```python
from build123d import *

# Parameters (mm, degrees)
F1_DEPTH      = 50
F1_DEPTH_BACK = 50
F2_T          = -5
F3_R          = 2.5
F4_DEPTH      = 5
F5_R          = 5
F5_R_2        = 2.5
F6_DEPTH      = 3


with BuildPart() as f1:
    # F0 (on Front) → F1 (new body, two sides)
    with BuildSketch(Plane.XZ) as f1_sk:
        Polygon((-50, 0), (50, 0), (60, 33.947153), (-60, 33.947153), align=None)
    extrude(amount=F1_DEPTH)
    extrude(f1_sk.sketch, amount=-F1_DEPTH_BACK)

    # F2
    f2_openings = [f1.faces().sort_by_distance(p)[0] for p in [
        (0, 0, 33.947153),
    ]]
    offset(amount=F2_T, openings=f2_openings)

    # F3 (on face) → F4 (cut, through all)
    with BuildSketch(Plane.XY.offset(5)):
        with Locations((-40, 40)):
            Circle(F3_R)
        with Locations((-40, -40)):
            Circle(F3_R)
        with Locations((40, -40)):
            Circle(F3_R)
        with Locations((40, 40)):
            Circle(F3_R)
    extrude(amount=-F4_DEPTH, mode=Mode.SUBTRACT)

    # F5 (on face) → F6 (cut)
    with BuildSketch(Plane(origin=(0, 0, 0), x_dir=(1, 0, 0), z_dir=(0, 0, -1))):
        with Locations((-40, 40)):
            Circle(F5_R)
        with Locations((-40, 40)):
            Circle(F5_R_2, mode=Mode.SUBTRACT)
        with Locations((40, 40)):
            Circle(F5_R)
        with Locations((40, 40)):
            Circle(F5_R_2, mode=Mode.SUBTRACT)
        with Locations((40, -40)):
            Circle(F5_R)
        with Locations((40, -40)):
            Circle(F5_R_2, mode=Mode.SUBTRACT)
        with Locations((-40, -40)):
            Circle(F5_R)
        with Locations((-40, -40)):
            Circle(F5_R_2, mode=Mode.SUBTRACT)
    extrude(amount=-F6_DEPTH, mode=Mode.SUBTRACT)


solid = f1.part
```
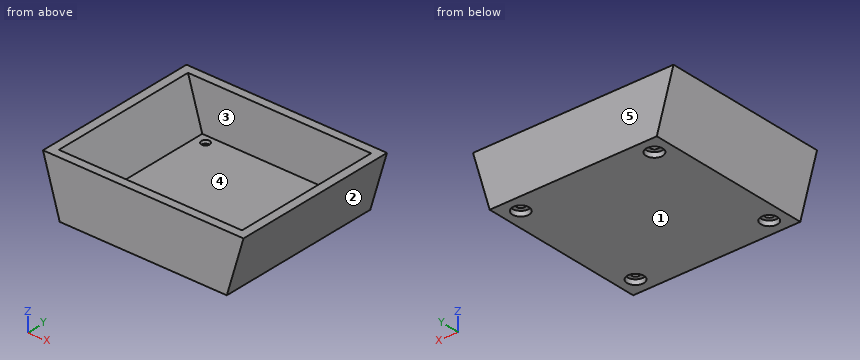
Geometry check sheet. Reference: the model listing, model coordinates, mm. Face numbers are marked on the shaded views. A direction names the side the tool comes from. Coordinates: 2 decimals unless noted, no trailing zeros. Order: outer loops, then holes, each group sorted by start corner. A loop starts at its lowest first (then second) coordinate and runs counter-clockwise, first axis right, second up.
Q1. Sectioned sample at D-D on x = -17.5. Record the cut outline in (y, z).
Reply:
outline: (-50, 0) - (50, 0) - (50, 33.95) - (45, 33.95) - (45, 5) - (-45, 5) - (-45, 33.95) - (-50, 33.95) - close
Q2. Sectioned sample at C-C on z = 28.5. Record the cut outline in (x, y).
Reply:
outline: (-58.4, -50) - (58.4, -50) - (58.4, 50) - (-58.4, 50) - close; hole (-53.18, -45) - (53.18, -45) - (53.18, 45) - (-53.18, 45) - close
Q3. Tool access check on the marked faces 4 and 5. Record the directions out of +Z, -Z, +X, -X, +Y, -Y that give a thin tool (end or side, any length) a straight path to the whole face; none if there is none.
Reply:
face 4: +Z
face 5: +Z, -Z, +X, -X, +Y
Q4. Sectioned sample at B-B on y = -40. Record the cut outline in (x, z).
Reply:
outline: (-60, 33.95) - (-50, 0) - (-45, 0) - (-45, 3) - (-42.5, 3) - (-42.5, 5) - (-46.26, 5) - (-54.79, 33.95) - close; (-37.5, 3) - (-35, 3) - (-35, 0) - (35, 0) - (35, 3) - (37.5, 3) - (37.5, 5) - (-37.5, 5) - close; (42.5, 3) - (45, 3) - (45, 0) - (50, 0) - (60, 33.95) - (54.79, 33.95) - (46.26, 5) - (42.5, 5) - close
Q5. Sectioned sample at A-A on x = 40. Record the cut outline in (y, z).
Reply:
outline: (-50, 0) - (-45, 0) - (-45, 3) - (-42.5, 3) - (-42.5, 5) - (-45, 5) - (-45, 33.95) - (-50, 33.95) - close; (-37.5, 3) - (-35, 3) - (-35, 0) - (35, 0) - (35, 3) - (37.5, 3) - (37.5, 5) - (-37.5, 5) - close; (42.5, 3) - (45, 3) - (45, 0) - (50, 0) - (50, 33.95) - (45, 33.95) - (45, 5) - (42.5, 5) - close
Q6. Depth check by flat-ended pin: pin 1 Ø12 at (y, z) = (10.5, 25.5) entering from -X; pin 2 Ø5 at (x, y) = (-41.5, 41) entering from -Z; pin 3 Ø12 at (y, z) = (-10.5, 24.5) entering from +X. Enter the tip coordinate at first touch or a pass-through.
Reply:
pin 1: stops at x = -59.28
pin 2: stops at z = 3
pin 3: stops at x = 58.98
Q7. Thickness scan on probe 1 along Y at (x, z) = (-40, 3.4); probe 2 along Y at (x, z) = (-40, 1.05); probe 3 along Y at (x, z) = (-46, 26.5). Record the ranges inside material, lowest first.
Reply:
probe 1: y = -50 to -42.5, -37.5 to 37.5, 42.5 to 50
probe 2: y = -50 to -45, -35 to 35, 45 to 50
probe 3: y = -50 to -45, 45 to 50
Q8. Draft check along X on the marked faces 1, 2 and 3. Enter one of: released by +X, released by -X, zero draft, split by the parting line, or undercut.
Reply:
face 1: zero draft
face 2: released by +X
face 3: undercut
